from build123d import *
from build123d.topology import SkipClean

# Parameters (mm, degrees)
SKETCH1_W           = 218.44
SKETCH1_H           = 12.7
BOSS_EXTRUDE1_DEPTH = 1.5875
BOSS_EXTRUDE3_DEPTH = 6.35
SKETCH3_R           = 3.175
BOSS_EXTRUDE4_DEPTH = 25.4
SKETCH5_R           = 3.175
BOSS_EXTRUDE5_DEPTH = 5.842
BOSS_EXTRUDE6_START = 5.842
SKETCH6_R           = 3.175
BOSS_EXTRUDE6_DEPTH = 5.842


with BuildPart() as part:
    # Sketch1 → Boss-Extrude1 (new, symmetric)
    with BuildSketch(Plane(origin=(0, 0, 0), x_dir=(1, 0, 0), z_dir=(0, 1, 0))):
        Rectangle(SKETCH1_W, SKETCH1_H)
    extrude(amount=BOSS_EXTRUDE1_DEPTH, both=True)

    # Sketch2 → Boss-Extrude3 (add)
    with BuildSketch(Plane(origin=(109.22, 0, 0), x_dir=(0, 0, -1), z_dir=(1, 0, 0))):
        with BuildLine():
            Line((-6.35, 3.175), (-51.054, 3.175))
            ThreePointArc((-51.054, 3.175), (-54.229, 0), (-51.054, -3.175))
            Line((-51.054, -3.175), (-6.35, -3.175))
            Line((-6.35, -3.175), (32.258, -3.175))
            ThreePointArc((32.258, -3.175), (35.433, 0), (32.258, 3.175))
            Line((32.258, 3.175), (-6.35, 3.175))
        make_face()
    boss_extrude3 = extrude(amount=BOSS_EXTRUDE3_DEPTH)

    # Sketch3 → Boss-Extrude4 (add)
    with SkipClean():  # the faces are left unmerged after this step: merging them gives an invalid solid
        with BuildSketch(Plane(origin=(115.57, 0, 0), x_dir=(0, 0, -1), z_dir=(1, 0, 0))):
            with Locations(Location((-51.054, 0, 0), (0, 0, 270))):
                Circle(SKETCH3_R)
        boss_extrude4 = extrude(amount=BOSS_EXTRUDE4_DEPTH)

    # Sketch5 → Boss-Extrude5 (add)
    with BuildSketch(Plane(origin=(115.57, 0, 0), x_dir=(0, 0, -1), z_dir=(1, 0, 0))):
        with Locations(Location((32.258, 0, 0), (0, 0, 90))):
            Circle(SKETCH5_R)
    boss_extrude5 = extrude(amount=BOSS_EXTRUDE5_DEPTH)

    # Sketch6 → Boss-Extrude6 (add)
    with BuildSketch(Plane.ZY.offset(-109.22).offset(BOSS_EXTRUDE6_START)):
        with Locations((-32.258, 0)):
            Circle(SKETCH6_R)
    boss_extrude6 = extrude(amount=-BOSS_EXTRUDE6_DEPTH)

    # Mirror1: Boss-Extrude3, Boss-Extrude4, Boss-Extrude5, Boss-Extrude6 across plane
    with SkipClean():  # the faces are left unmerged after this step: merging them gives an invalid solid
        add(boss_extrude3.mirror(Plane(origin=(0, 0, 0), x_dir=(0, 0, 1), z_dir=(1, 0, 0))))
        add(boss_extrude4.mirror(Plane(origin=(0, 0, 0), x_dir=(0, 0, 1), z_dir=(1, 0, 0))))
        add(boss_extrude5.mirror(Plane(origin=(0, 0, 0), x_dir=(0, 0, 1), z_dir=(1, 0, 0))))
        add(boss_extrude6.mirror(Plane(origin=(0, 0, 0), x_dir=(0, 0, 1), z_dir=(1, 0, 0))))
    add(part.part.scale(1), mode=Mode.REPLACE)  # the faces are merged on a copy


solid = part.part
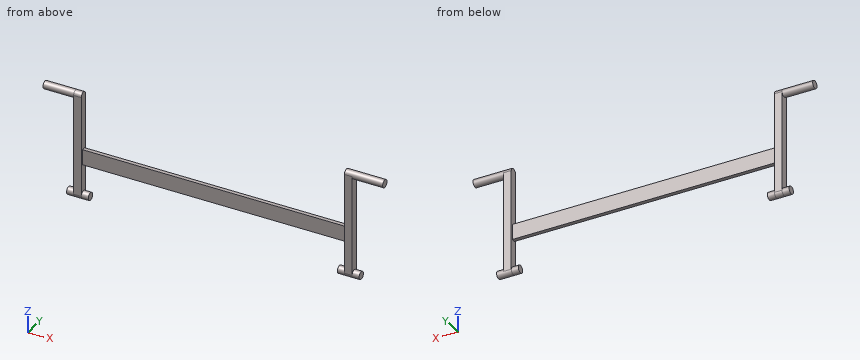
The model under review builds one solid part; all positions refer to its coordinate system, in mm. Coordinates: 2 decimals unless noted, no trailing zeros. Write each loop counter-clockwise with the first axis right and the second up, starting at its lowest first coordinate (ties: lowest second). Pieces come first, ordered by that corner, then holes. Notation, with made-up numbers: (-34.5, 16.25) - (8.5, 16.25) arc R14 ccw to (8.5, 40.25) - close; hole circle Ø4 at (88.25, -6.5). An arc over 180 degrees is marked (long way). Answer as CSV lines item,"result".
(1) We need section A-A (z = 32). Give the boundary of the cut face in (x, y) (3 decimals).
Data:
outline,"(-115.57, -3.175) - (-109.22, -3.175) - (-109.22, 3.175) - (-115.57, 3.175) - close; (109.22, -3.175) - (115.57, -3.175) - (115.57, 3.175) - (109.22, 3.175) - close"
(2) Clearance check with flat-ended pins moving along their axes: pin 1 Ø10 at (x, z) = (-13, 2) entering from -Y; pin 2 Ø2.5 at (x, y) = (45.5, 0.5) entering from +Z; pin 3 Ø1.6 at (x, y) = (-49, 0) entering from -Z. State where each tip first meets the part, or that it passes through.
Data:
pin 1,"stops at y = -1.59"
pin 2,"stops at z = 6.35"
pin 3,"stops at z = -6.35"
(3) For line 1 along X through (y, z) = (-1, -8); line 2 along X through (y, z) = (1.5, -6); line 3 along X through (y, z) = (-0.75, -30), list the stretches that pass through material, from the lowest coordinate up. Write a range as [from, to].
Data:
line 1,"x = [-115.57, -109.22], [109.22, 115.57]"
line 2,"x = [-115.57, 115.57]"
line 3,"x = [-121.41, -103.38], [103.38, 121.41]"
(4) We need section B-B (x = -71.5). Give the boundary of the cut face in (y, z).
Data:
outline,"(-1.59, -6.35) - (1.59, -6.35) - (1.59, 6.35) - (-1.59, 6.35) - close"
